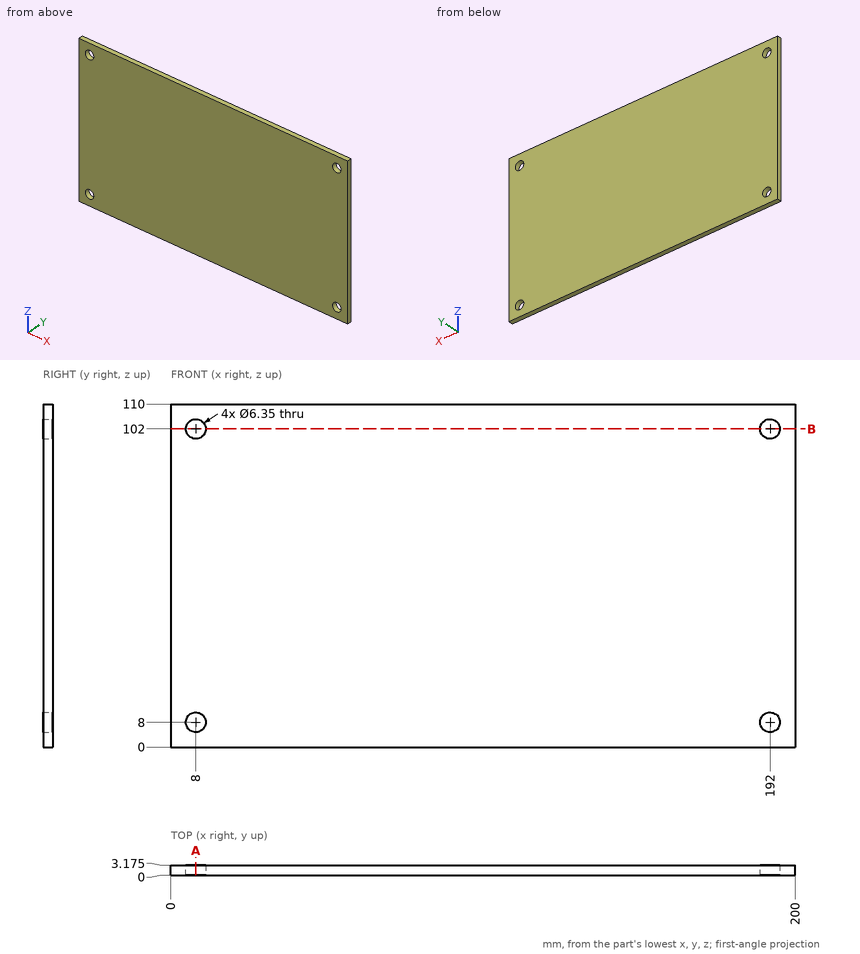
For this review, use the dimensioned drawing (mm, ordinates from the lowest corner) and the shaded views. Coordinates: 2 decimals unless noted, no trailing zeros. Write each loop counter-clockwise with the first axis right and the second up, starting at its lowest first coordinate (ties: lowest second). Pieces come first, ordered by that corner, then holes. Notation, with made-up numbers: (-12.75, -8.75) -> (22.25, -8.75) arc R22 cw to (22.25, 10.25) -> close; hole circle Ø10 at (48, -27). An arc over 180 degrees is marked (long way). Put each result on its own line as item: value.
Q1. Take a section at A-A, the plane x = 8. State the section outline as (y, z) points (3 decimals), then the cut area to 3 significant figures.
From the geometry:
outline: (0, 0) -> (3.175, 0) -> (3.175, 4.825) -> (0, 4.825) -> close; (0, 11.175) -> (3.175, 11.175) -> (3.175, 98.825) -> (0, 98.825) -> close; (0, 105.175) -> (3.175, 105.175) -> (3.175, 110) -> (0, 110) -> close
area: 309 mm2
Q2. Clearance check with a flat-ended pin moving along its axis: pin 1 Ø5.5 at (x, z) = (192, 8) entering from -Y. State where the tip first meets the part, or that it passes through.
From the geometry:
pin 1: passes through
Q3. Wall thickness on L1, parallel to X at y = 0.4, z = 101.5; L2, parallel to X at y = 1.25, z = 8 (3 decimals); L3, parallel to Z at x = 8, y = 2.45 (3 decimals): over which ranges is each line inside the solid? List them lowest first.
From the geometry:
L1: x = 0 to 4.86, 11.14 to 188.86, 195.14 to 200
L2: x = 0 to 4.825, 11.175 to 188.825, 195.175 to 200
L3: z = 0 to 4.825, 11.175 to 98.825, 105.175 to 110
Q4. Take a section at B-B, the plane z = 102. State the section outline as (x, y) points (3 decimals).
From the geometry:
outline: (0, 0) -> (4.825, 0) -> (4.825, 3.175) -> (0, 3.175) -> close; (11.175, 0) -> (188.825, 0) -> (188.825, 3.175) -> (11.175, 3.175) -> close; (195.175, 0) -> (200, 0) -> (200, 3.175) -> (195.175, 3.175) -> close
